Input: dimensioned drawing with shaded views. Units: mm. Origin: part minimum x, y, z. A direction names the side the tool comes from. Round coordinates to 2 decimals unless told otherwise and drop trailing zeros. Loops run counter-clockwise (first coordinate to the right, second up) from the corner with the lowest first, then second, coordinate; pieces in that order, holes last. Notation, with made-up numbers: (-12.5, 54.5) -> (20.5, 54.5) arc R12 ccw to (20.5, 71.5) -> close; hole circle Ø8 at (-24.5, 39). An arc over 180 degrees is marked (long way). Answer as a JSON object with one key per item and string values.
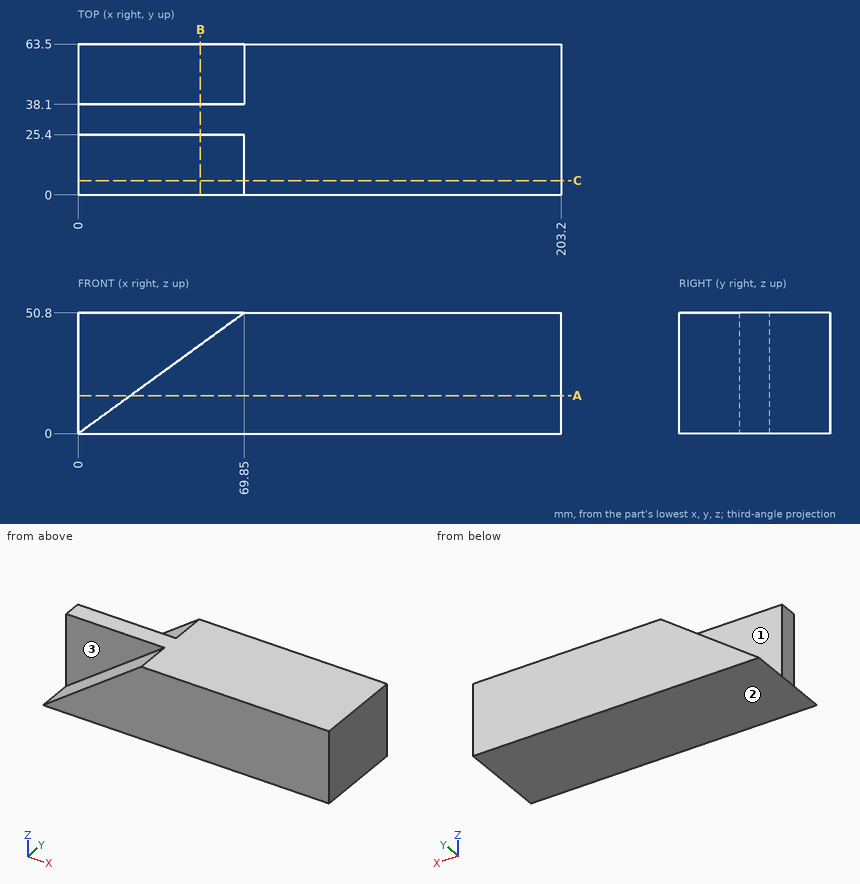
1) Section B-B, the plane x = 51.5. Output: boundary loops of the cut face in (y, z).
Output:
{"outline": "(0, 0) -> (63.5, 0) -> (63.5, 37.45) -> (38.1, 37.45) -> (38.1, 50.8) -> (25.4, 50.8) -> (25.4, 37.45) -> (0, 37.45) -> close"}
2) Section C-C, the plane y = 6. Output: boundary loops of the cut face in (x, z).
Output:
{"outline": "(0, 0) -> (203.2, 0) -> (203.2, 50.8) -> (69.85, 50.8) -> close"}
3) Contact query for flat-ended pins moving along their axis: P1, Ø2, axis at y = 17.5, z = 25, coming from the -X side; P2, Ø3, axis at x = 34.5, y = 44, coming from the +Z side. Output: stop coordinate, or through.
Output:
{"P1": "stops at x = 33", "P2": "stops at z = 26.18"}
4) Section A-A, the plane z = 16. Output: boundary loops of the cut face in (x, y), plus the area to 3 significant figures.
Output:
{"outline": "(0, 25.4) -> (22, 25.4) -> (22, 0) -> (203.2, 0) -> (203.2, 63.5) -> (22, 63.5) -> (22, 38.1) -> (0, 38.1) -> close", "area": "11,800 mm^2"}
5) Reachability of the marked faces 1, 2 and 3 from +Z, -Z, +X, -X, +Y, -Y: full face, straight path, thin tool, end or side. Return the list, or none.
Output:
{"face 1": "+Z, -X, +Y", "face 2": "-Z, +X, -X, +Y, -Y", "face 3": "+Z, -X, -Y"}
6) Ray query, probe 1 along Y at (x, z) = (40, 45); probe 2 along Z at (x, y) = (16, 45.5); probe 3 along X at (y, z) = (6, 13) (3 decimals). Return the intervals inside material, ascending.
Output:
{"probe 1": "y = 25.4 to 38.1", "probe 2": "z = 0 to 11.64", "probe 3": "x = 17.875 to 203.2"}
